```python
from build123d import *

# Parameters (mm, degrees)
F0_W           = 35
F0_H           = 35
F1_DEPTH       = 5
F2_R           = 3
F3_DEPTH       = 5.001
F5_D           = 3.3
F5_CBORE_D     = 6.5
F5_CBORE_DEPTH = 3
F6_SIZE        = 2.5
F7_R           = 1
F8_R           = 1.5
F9_DEPTH       = 5.001
F10_R          = 1.9
F11_DEPTH      = 4


with BuildPart() as f1:
    # F0 (on Front) → F1 (new body)
    with BuildSketch(Plane.XZ):
        Rectangle(F0_W, F0_H)
    extrude(amount=F1_DEPTH)

    # F2 (on face) → F3 (cut, through all)
    with BuildSketch(Plane.XZ.offset(5)):
        Circle(F2_R)
    extrude(amount=-F3_DEPTH, mode=Mode.SUBTRACT)

    # F5 (through all)
    with Locations(Plane.XZ.offset(5)):
        with Locations((-13, 13), (13, 13), (13, -13), (-13, -13)):
            CounterBoreHole(F5_D / 2, F5_CBORE_D / 2, F5_CBORE_DEPTH)

    # F6
    f6_edges = [f1.edges().sort_by_distance(p)[0] for p in [
        (17.5, -2.5, 17.5),
        (-17.5, -2.5, 17.5),
        (17.5, -2.5, -17.5),
        (-17.5, -2.5, -17.5),
    ]]
    chamfer(f6_edges, length=F6_SIZE)

    # F7
    f7_edges = [f1.edges().sort_by_distance(p)[0] for p in [
        (15, -2.5, 17.5),
        (17.5, -2.5, 15),
        (17.5, -2.5, -15),
        (15, -2.5, -17.5),
        (-15, -2.5, -17.5),
        (-17.5, -2.5, -15),
        (-15, -2.5, 17.5),
        (-17.5, -2.5, 15),
    ]]
    fillet(f7_edges, radius=F7_R)

    # F8 (on face) → F9 (cut, through all)
    with BuildSketch(Plane.XZ.offset(5)):
        with Locations((0, 9.525)):
            Circle(F8_R)
        with Locations((0, -9.525)):
            Circle(F8_R)
    extrude(amount=-F9_DEPTH, mode=Mode.SUBTRACT)

    # F10 (on face) → F11 (cut)
    with BuildSketch(Plane(origin=(0, 0, 0), x_dir=(-1, 0, 0), z_dir=(0, 1, 0))):
        with Locations((0, -9.525)):
            Circle(F10_R)
        with Locations((0, 9.525)):
            Circle(F10_R)
    extrude(amount=-F11_DEPTH, mode=Mode.SUBTRACT)


solid = f1.part
```
Source: CAD feature listing. Evaluate the final solid. Frame: model axes, mm. A direction names the side the tool comes from. Round coordinates to 2 decimals unless told otherwise and drop trailing zeros. Loops run counter-clockwise (first coordinate to the right, second up) from the corner with the lowest first, then second, coordinate; pieces in that order, holes last. Notation, with made-up numbers: M 64,62 L 103,62 A18 cw 103,91 Z; hole C 68.5,21.25 d5. An arc over 180 degrees is marked long. Use a Markdown table: item, result. Add a question column.
1. Ray query, line 1 along Z through (x, y) = (0, -4.6) (3 decimals); line 2 along Z through (x, y) = (13, -1.05); line 3 along Z through (x, y) = (0, -2.55) (3 decimals). Return the intervals inside material, ascending. Write a range as [from, to].
2. Contact query for flat-ended pins moving along their axis: pin 1 (1 mm diameter, centred on x = 2, z = 11, fed in from +Y); pin 2 (3.5 mm diameter, centred on x = 0, z = -9.525, fed in from +Y); pin 3 (5.5 mm diameter, centred on x = 13, z = -13, fed in from -Y). Output: stop coordinate, or through.
3. Cut plane C-C, the plane z = 0. Output: boundary loops of the cut face in (x, y).
4. Cut plane D-D, the plane y = -3.15. Output: boundary loops of the cut face in (x, z) (3 decimals), and give its area (3 significant figures).
5. Set-up query: faces 1 (the cylindrical face through (-1.02, -1.97, -7.92)), 2 (the cylindrical face through (-0.2, -4.51, -8.04)), 3 (the flat face through (14.4, -2, 11.6)). Return all of +Z, -Z, +X, -X, +Y, -Y with unobstructed straight access to the full face (end or side cutting, diameter ignored); none if empty.
6. Pull-direction query (Z, two-part tool) for faces 4 (the flat face through (-17.5, -2, 0)), 5 (the flat face through (16.3, -2.5, -16.2)), 6 (the cylindrical face through (-15.395, -3.521, -10.803)); classes: +Z half, -Z half, draft (parallel to the pull), parting line (faces both ways), or undercut.
7. Cut plane B-B, the plane x = -13. Output: boundary loops of the cut face in (y, z).
8. Cut plane A-A, the plane z = 13. Output: boundary loops of the cut face in (x, y), and give its area (3 significant figures).
Solution:
| question | item | result |
|---|---|---|
| 1 | line 1 | z = [-17.5, -11.025], [-8.025, -3], [3, 8.025], [11.025, 17.5] |
| 1 | line 2 | z = [-17.5, -14.65], [-11.35, 11.35], [14.65, 17.5] |
| 1 | line 3 | z = [-17.5, -11.425], [-7.625, -3], [3, 7.625], [11.425, 17.5] |
| 2 | pin 1 | stops at y = 0 |
| 2 | pin 2 | stops at y = -4 |
| 2 | pin 3 | stops at y = -2 |
| 3 | outline | M -17.5,-5 L -3,-5 L -3,0 L -17.5,0 Z; M 3,-5 L 17.5,-5 L 17.5,0 L 3,0 Z |
| 4 | outline | M -17.5,-14.586 A1 ccw -17.207,-15.293 L -15.293,-17.207 A1 ccw -14.586,-17.5 L 14.586,-17.5 A1 ccw 15.293,-17.207 L 17.207,-15.293 A1 ccw 17.5,-14.586 L 17.5,14.586 A1 ccw 17.207,15.293 L 15.293,17.207 A1 ccw 14.586,17.5 L -14.586,17.5 A1 ccw -15.293,17.207 L -17.207,15.293 A1 ccw -17.5,14.586 Z; hole C -13,-13 d6.5; hole C -13,13 d6.5; hole C 0,0 d6; hole C 0,-9.525 d3.8; hole C 0,9.525 d3.8; hole C 13,-13 d6.5; hole C 13,13 d6.5 |
| 4 | area | 1,030 mm2 |
| 5 | face 1 | +Y |
| 5 | face 2 | +Y, -Y |
| 5 | face 3 | -Y |
| 6 | face 4 | draft |
| 6 | face 5 | -Z half |
| 6 | face 6 | undercut |
| 7 | outline | M -5,-17.5 L 0,-17.5 L 0,-14.65 L -2,-14.65 L -2,-16.25 L -5,-16.25 Z; M -5,-9.75 L -2,-9.75 L -2,-11.35 L 0,-11.35 L 0,11.35 L -2,11.35 L -2,9.75 L -5,9.75 Z; M -5,16.25 L -2,16.25 L -2,14.65 L 0,14.65 L 0,17.5 L -5,17.5 Z |
| 8 | outline | M -17.5,-5 L -16.25,-5 L -16.25,-2 L -14.65,-2 L -14.65,0 L -17.5,0 Z; M -11.35,-2 L -9.75,-2 L -9.75,-5 L 9.75,-5 L 9.75,-2 L 11.35,-2 L 11.35,0 L -11.35,0 Z; M 14.65,-2 L 16.25,-2 L 16.25,-5 L 17.5,-5 L 17.5,0 L 14.65,0 Z |
| 8 | area | 123 mm2 |
